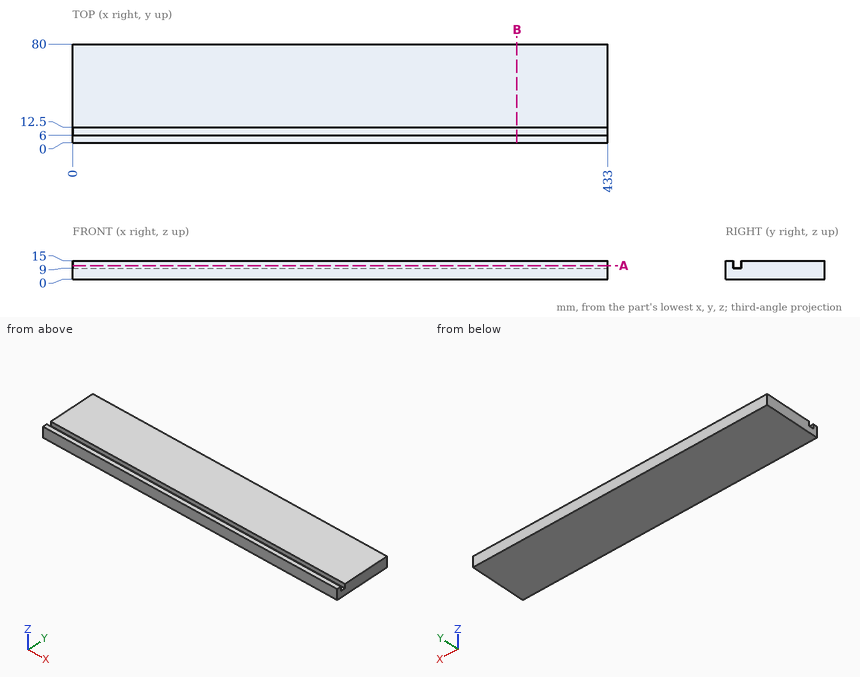
Drawing for the job (mm, zero at the part's lowest x, y, z). Give positions to 0.01 mm unless a question says otherwise; leave off trailing zeros. Write each loop counter-clockwise with the first axis right and the second up, starting at its lowest first coordinate (ties: lowest second). Pieces come first, ordered by that corner, then holes. Notation, with made-up numbers: M -1,16 L 6,16 A7 ccw 6,26 Z; hole C 15.5,20 d4. An arc over 180 degrees is marked long. Use CSV: the item, a comma, the result in double quotes.
Item 1: Slice it at B-B on x = 359.5. Write the cut outline in (y, z), plus the area to 3 significant figures.
Taken from the geometry:
outline,"M 0,0 L 80,0 L 80,15 L 12.5,15 L 12.5,9 L 6,9 L 6,15 L 0,15 Z"
area,"1,160 mm²"
Item 2: Drill centre lines: probe 1 along Y at (x, z) = (269, 11.5); probe 2 along Z at (x, y) = (299.5, 8). Where is each one in solid material? Low to high.
Taken from the geometry:
probe 1,"y = 0 to 6, 12.5 to 80"
probe 2,"z = 0 to 9"
Item 3: Pin check, flat tip, straight feed: P1, Ø2, axis at y = 10.5, z = 13.5, coming from the -X side. Stop position of the tip, or through.
Taken from the geometry:
P1,"passes through"
Item 4: Slice it at A-A on z = 11.25. Write the cut outline in (x, y), plus the area to 3 significant figures.
Taken from the geometry:
outline,"M 0,0 L 433,0 L 433,6 L 0,6 Z; M 0,12.5 L 433,12.5 L 433,80 L 0,80 Z"
area,"31,800 mm²"
